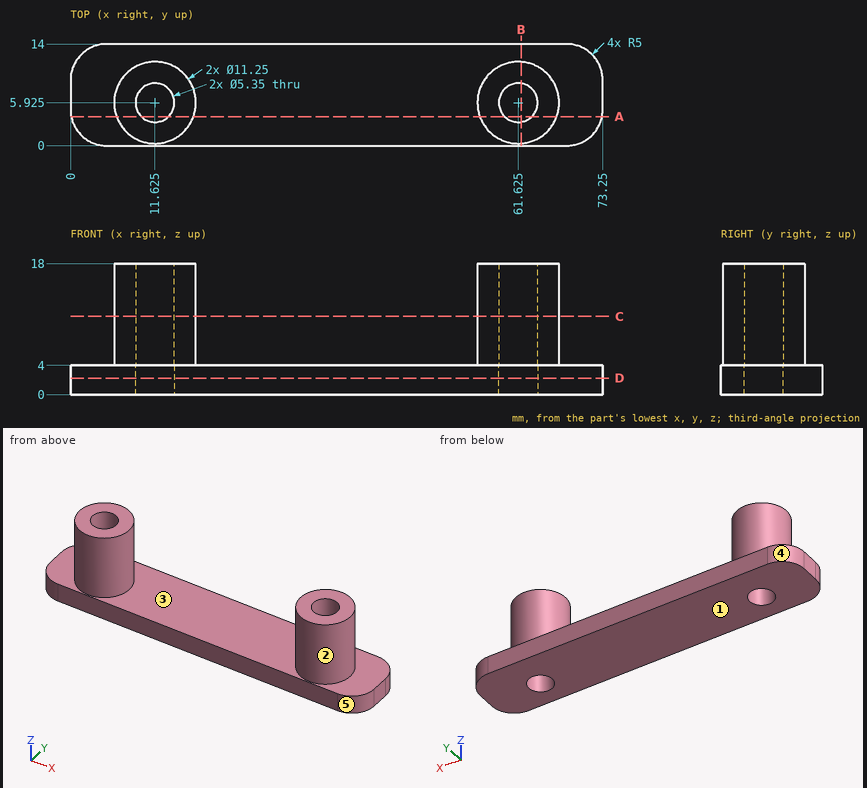
Source: three-view drawing plus pictorial views. Frame: mm from the lowest corner of the part. A direction names the side the tool comes from. Round coordinates to 2 decimals unless told otherwise and drop trailing zeros. Loops run counter-clockwise (first coordinate to the right, second up) from the corner with the lowest first, then second, coordinate; pieces in that order, holes last. Notation, with made-up numbers: M 15.5,68 L 26.5,68 A31 ccw 26.5,100 Z; hole C 78.5,-8.75 d9. An arc over 180 degrees is marked long. Answer as CSV lines item,"result". Start each with the question number.
(1) Section C-C, the plane z = 10.75. Output: boundary loops of the cut face in (x, y) (3 decimals).
(2) First-contact query: pin 1 (4 mm diameter, centred on y = 10, z = 9, fed in from +X); pin 2 (5 mm diameter, centred on y = 11, z = 13, fed in from -X); pin 3 (3 mm diameter, centred on y = 11, z = 8, fed in from +X). Flat tips, straight axial feed; report the tip coordinate or a pass-through.
(3) Section A-A, the plane y = 4. Output: boundary loops of the cut face in (x, z), plus the area to 3 significant figures.
(4) Reachability of the marked faces 1 and 2 from +Z, -Z, +X, -X, +Y, -Y: full face, straight path, thin tool, end or side. Return the list, or none.
(5) Section D-D, the plane z = 2.25. Output: boundary loops of the cut face in (x, y) (3 decimals), plus the area to 3 significant figures.
(6) Line query: line 1 (X direction, y = 6.25, z = 6.25); line 2 (Z direction, x = 5.5, y = 8.5); line 3 (X direction, y = 5, z = 10.75). Output: solid intervals per line, ascending. Write a range as [from, to].
(7) Draft query along X for the marked faces 3, 4 and 5. Return one class per face: released by +X, released by -X, zero draft, split by the parting line, or undercut.
(8) Section B-B, the plane x = 62. Output: boundary loops of the cut face in (y, z).
Values found:
1,outline,"C 11.625,5.925 d11.25; C 61.625,5.925 d11.25; hole C 11.625,5.925 d5.35; hole C 61.625,5.925 d5.35"
2,pin 1,"stops at x = 66.85"
2,pin 2,"stops at x = 6.62"
2,pin 3,"stops at x = 65.97"
3,outline,"M 0.1,0 L 9.77,0 L 9.77,18 L 6.34,18 L 6.34,4 L 0.1,4 Z; M 13.48,0 L 59.77,0 L 59.77,18 L 56.34,18 L 56.34,4 L 16.91,4 L 16.91,18 L 13.48,18 Z; M 63.48,0 L 73.15,0 L 73.15,4 L 66.91,4 L 66.91,18 L 63.48,18 Z"
3,area,"454 mm²"
4,face 1,"-Z, +X, -X, +Y, -Y"
4,face 2,"+Z"
5,outline,"M 0,5 A5 ccw 5,0 L 68.25,0 A5 ccw 73.25,5 L 73.25,9 A5 ccw 68.25,14 L 5,14 A5 ccw 0,9 Z; hole C 11.625,5.925 d5.35; hole C 61.625,5.925 d5.35"
5,area,"959 mm²"
6,line 1,"x = [6.01, 8.97], [14.28, 17.24], [56.01, 58.97], [64.28, 67.24]"
6,line 2,"z = [0, 4]"
6,line 3,"x = [6.08, 9.12], [14.13, 17.17], [56.08, 59.12], [64.13, 67.17]"
7,face 3,"undercut"
7,face 4,"released by -X"
7,face 5,"released by +X"
8,outline,"M 0,0 L 3.28,0 L 3.28,18 L 0.31,18 L 0.31,4 L 0,4 Z; M 8.57,0 L 14,0 L 14,4 L 11.54,4 L 11.54,18 L 8.57,18 Z"
